```python
from build123d import *

# Parameters (mm, degrees)
SKETCH1_R           = 2
SKETCH1_R_2         = 3.4
SKETCH1_R_3         = 5.65
BOSS_EXTRUDE1_DEPTH = 20
SKETCH2_W           = 52
SKETCH2_H           = 44
SKETCH2_H_2         = 75
CUT_EXTRUDE1_DEPTH  = 15


with BuildPart() as part:
    # Sketch1 → Boss-Extrude1 (new body)
    with BuildSketch(Plane(origin=(0, 0, 0), x_dir=(1, 0, 0), z_dir=(0, 1, 0))):
        Polygon((26, -118.035), (26, -162.035), (-26, -162.035), (-26, -118.035), (-37.625, -118.035), (-37.625, 118.035), (-26, 118.035), (-26, 193.035), (26, 193.035), (26, 118.035), (37.625, 118.035), (37.625, -118.035), align=None)
        with Locations(Location((-21, -123.035, 0), (0, 0, 270))):
            Circle(SKETCH1_R, mode=Mode.SUBTRACT)
        with Locations(Location((21, -123.035, 0), (0, 0, 270))):
            Circle(SKETCH1_R, mode=Mode.SUBTRACT)
        with Locations(Location((-21, -157.035, 0), (0, 0, 270))):
            Circle(SKETCH1_R, mode=Mode.SUBTRACT)
        with Locations(Location((21, -157.035, 0), (0, 0, 270))):
            Circle(SKETCH1_R, mode=Mode.SUBTRACT)
        with Locations(Location((15, 188.035, 0), (0, 0, 270))):
            Circle(SKETCH1_R_2, mode=Mode.SUBTRACT)
        with Locations(Location((-15, 188.035, 0), (0, 0, 270))):
            Circle(SKETCH1_R_2, mode=Mode.SUBTRACT)
        with Locations(Location((15, 129.035, 0), (0, 0, 270))):
            Circle(SKETCH1_R_2, mode=Mode.SUBTRACT)
        with Locations(Location((-15, 129.035, 0), (0, 0, 270))):
            Circle(SKETCH1_R_2, mode=Mode.SUBTRACT)
        with Locations(Location((-22.995, 103.115, 0), (0, 0, 270))):
            Circle(SKETCH1_R_3, mode=Mode.SUBTRACT)
        with Locations(Location((0.005, 103.115, 0), (0, 0, 270))):
            Circle(SKETCH1_R_3, mode=Mode.SUBTRACT)
        with Locations(Location((23.005, 103.115, 0), (0, 0, 270))):
            Circle(SKETCH1_R_3, mode=Mode.SUBTRACT)
        with Locations(Location((0.005, 83.115, 0), (0, 0, 270))):
            Circle(SKETCH1_R_3, mode=Mode.SUBTRACT)
        with Locations(Location((23.005, 83.115, 0), (0, 0, 270))):
            Circle(SKETCH1_R_3, mode=Mode.SUBTRACT)
        with Locations(Location((0.005, 63.115, 0), (0, 0, 270))):
            Circle(SKETCH1_R_3, mode=Mode.SUBTRACT)
        with Locations(Location((23.005, 63.115, 0), (0, 0, 270))):
            Circle(SKETCH1_R_3, mode=Mode.SUBTRACT)
        with Locations(Location((0.005, 43.115, 0), (0, 0, 270))):
            Circle(SKETCH1_R_3, mode=Mode.SUBTRACT)
        with Locations(Location((23.005, 43.115, 0), (0, 0, 270))):
            Circle(SKETCH1_R_3, mode=Mode.SUBTRACT)
        with Locations(Location((0.005, 23.115, 0), (0, 0, 270))):
            Circle(SKETCH1_R_3, mode=Mode.SUBTRACT)
        with Locations(Location((23.005, 23.115, 0), (0, 0, 270))):
            Circle(SKETCH1_R_3, mode=Mode.SUBTRACT)
        with Locations(Location((0.005, 3.115, 0), (0, 0, 270))):
            Circle(SKETCH1_R_3, mode=Mode.SUBTRACT)
        with Locations(Location((23.005, 3.115, 0), (0, 0, 270))):
            Circle(SKETCH1_R_3, mode=Mode.SUBTRACT)
        with Locations(Location((0.005, -16.885, 0), (0, 0, 270))):
            Circle(SKETCH1_R_3, mode=Mode.SUBTRACT)
        with Locations(Location((23.005, -16.885, 0), (0, 0, 270))):
            Circle(SKETCH1_R_3, mode=Mode.SUBTRACT)
        with Locations(Location((0.005, -36.885, 0), (0, 0, 270))):
            Circle(SKETCH1_R_3, mode=Mode.SUBTRACT)
        with Locations(Location((23.005, -36.885, 0), (0, 0, 270))):
            Circle(SKETCH1_R_3, mode=Mode.SUBTRACT)
        with Locations(Location((0.005, -56.885, 0), (0, 0, 270))):
            Circle(SKETCH1_R_3, mode=Mode.SUBTRACT)
        with Locations(Location((23.005, -56.885, 0), (0, 0, 270))):
            Circle(SKETCH1_R_3, mode=Mode.SUBTRACT)
        with Locations(Location((-22.995, 83.115, 0), (0, 0, 270))):
            Circle(SKETCH1_R_3, mode=Mode.SUBTRACT)
        with Locations(Location((-22.995, 63.115, 0), (0, 0, 270))):
            Circle(SKETCH1_R_3, mode=Mode.SUBTRACT)
        with Locations(Location((-22.995, 43.115, 0), (0, 0, 270))):
            Circle(SKETCH1_R_3, mode=Mode.SUBTRACT)
        with Locations(Location((-22.995, 23.115, 0), (0, 0, 270))):
            Circle(SKETCH1_R_3, mode=Mode.SUBTRACT)
        with Locations(Location((-22.995, 3.115, 0), (0, 0, 270))):
            Circle(SKETCH1_R_3, mode=Mode.SUBTRACT)
        with Locations(Location((-22.995, -16.885, 0), (0, 0, 270))):
            Circle(SKETCH1_R_3, mode=Mode.SUBTRACT)
        with Locations(Location((-22.995, -36.885, 0), (0, 0, 270))):
            Circle(SKETCH1_R_3, mode=Mode.SUBTRACT)
        with Locations(Location((-22.995, -56.885, 0), (0, 0, 270))):
            Circle(SKETCH1_R_3, mode=Mode.SUBTRACT)
    extrude(amount=BOSS_EXTRUDE1_DEPTH)

    # Sketch2 → Cut-Extrude1 (cut)
    with BuildSketch(Plane(origin=(0, 20, 0), x_dir=(1, 0, 0), z_dir=(0, 1, 0))):
        with Locations((0, -140.035)):
            Rectangle(SKETCH2_W, SKETCH2_H)
        with Locations((0, 155.535)):
            Rectangle(SKETCH2_W, SKETCH2_H_2)
    extrude(amount=-CUT_EXTRUDE1_DEPTH, mode=Mode.SUBTRACT)


solid = part.part
```
The listing builds one solid part. Answer for the finished solid, in the listing's coordinates (mm). Coordinates: 2 decimals unless noted, no trailing zeros. Write each loop counter-clockwise with the first axis right and the second up, starting at its lowest first coordinate (ties: lowest second). Pieces come first, ordered by that corner, then holes.
Q1. Section A-A, the plane y = 12.25 is taken. Give the number of separate pieces and of enclosed holes in the cut face, then the cut area to 3 significant figures.
Returned:
separate pieces: 1
enclosed holes: 27
area: 15,100 mm2
Q2. Section B-B, the plane x = 32 is taken. Write down the section's boundary in (y, z) (3 decimals).
Returned:
outline: (0, -118.035) - (20, -118.035) - (20, 118.035) - (0, 118.035) - close
Q3. The mould has two halves that part along X. Classify faces 1 (the cylindrical face through (17.49, 9.86, 35.66)), 2 (the flat face through (37.625, 10, -2)), 3 (the flat face through (0, 5, -156)): released by +X, released by -X, zero draft, split by the parting line, or undercut.
Returned:
face 1: undercut
face 2: released by +X
face 3: zero draft
Q4. Given P1, Ø5, axis at x = -7, y = 14.5, coming from the +Z side (3 decimals); P2, Ø15.5, axis at x = -8, z = -143, coming from the +Y side; P3, Ø2.5, axis at y = 3, z = 133.5, coming from the -X side, each flat-ended and moving along its own axis, determine where each tip first touches the part or whether it passes through.
Returned:
P1: stops at z = 118.035
P2: stops at y = 5
P3: stops at x = -26
Q5. Find the intervals of material crossed by line 1 along Z through (x, y) = (15, 3.2) (3 decimals); line 2 along X through (y, z) = (7, -43.5) (3 decimals); line 3 along X through (y, z) = (6.5, -22) (3 decimals), in increasing order.
Returned:
line 1: z = -193.035 to -191.435, -184.635 to -132.435, -125.635 to 162.035
line 2: x = -37.625 to -28.632, -17.358 to -5.632, 5.642 to 17.368, 28.642 to 37.625
line 3: x = -37.625 to -28.534, -17.456 to -5.534, 5.544 to 17.466, 28.544 to 37.625
